Input: part model. Units: mm. Frame: model coordinates. Give positions to 0.01 mm unless a question says otherwise; leave off trailing zeros. Loops run counter-clockwise (first coordinate to the right, second up) from the corner with the lowest first, then second, coordinate; pieces in that order, holes last. Notation, with made-up numbers: M -33,-28 L 7,-28 A21 ccw 7,11 Z; hole C 49.25,77 d4. An arc over 180 degrees is marked long. One line per item, written item: value. Start each with the question number.
(1) Pin query (flat end, axial travel): P1, Ø1.1, axis at x = -2.5, z = 2, coming from the +Y side; P2, Ø1.5, axis at x = 206, z = 4, coming from the -Y side. Return the tip coordinate at first contact, or that it passes through.
(2) Ray query, line 1 along X through (y, z) = (-26.5, 2); line 2 along X through (y, z) = (41, 1); line 3 along X through (y, z) = (13, 1) (1 decimal). Return the intervals inside material, ascending. Write a range as from..to.
(3) Section A-A on z = 3. State how many separate pieces and enclosed holes the cut face has, plus the area to 3 significant figures.
(4) Section B-B on y = 57.5. Output: boundary loops of the cut face in (x, z).
```python
from build123d import *

# Parameters (mm, degrees)
SKETCH1_W             = 393.065
SKETCH1_H             = 127
BOSS_EXTRUDE1_DEPTH   = 6.35
SKETCH2_W             = 76.2
SKETCH2_H             = 25.654
CUT_EXTRUDE1_DEPTH    = 6.35
CUT_EXTRUDE2_DEPTH    = 6.35
LPATTERN1_COUNT       = 5
LPATTERN1_PITCH       = 22.225
BOSS_EXTRUDE2_DEPTH   = 6.35
LPATTERN2_COUNT       = 5
LPATTERN2_PITCH       = 22.225
BOSS_EXTRUDE3_DEPTH   = 6.35
BOSS_EXTRUDE3_2_DEPTH = 6.35
LPATTERN4_COUNT       = 3
LPATTERN4_PITCH       = 111.252
SKETCH14_W            = 50.8
SKETCH14_H            = 6.35
CUT_EXTRUDE3_DEPTH    = 6.35
SKETCH16_W            = 50.8
SKETCH16_H            = 6.35
CUT_EXTRUDE4_DEPTH    = 6.35
SKETCH19_W            = 47.8155
SKETCH19_H            = 6.35
CUT_EXTRUDE5_DEPTH    = 6.35


with BuildPart() as part:
    # Sketch1 → Boss-Extrude1 (new body)
    with BuildSketch(Plane.XY):
        Rectangle(SKETCH1_W, SKETCH1_H)
    extrude(amount=BOSS_EXTRUDE1_DEPTH)

    # Sketch2 → Cut-Extrude1 (cut)
    with BuildSketch(Plane.XY.offset(6.35)):
        with Locations((2.7305, -25.273)):
            Rectangle(SKETCH2_W, SKETCH2_H)
    extrude(amount=-CUT_EXTRUDE1_DEPTH, mode=Mode.SUBTRACT)

    # Sketch3 → Cut-Extrude2 (cut)
    with BuildSketch(Plane.XY.offset(6.35)):
        Polygon((-196.5325, 47.625), (-190.1825, 47.625), (-190.1825, 51.181), (-185.1025, 51.181), (-185.1025, 37.719), (-190.1825, 37.719), (-190.1825, 41.275), (-196.5325, 41.275), align=None)
    cut_extrude2 = extrude(amount=-CUT_EXTRUDE2_DEPTH, mode=Mode.SUBTRACT)

    # LPattern1: Cut-Extrude2 ×5
    with Locations(*[(0, -i * LPATTERN1_PITCH, 0) for i in range(1, LPATTERN1_COUNT)]):
        add(cut_extrude2, mode=Mode.SUBTRACT)


with BuildPart() as body_2:
    # Sketch4 → Boss-Extrude2 (new body)
    with BuildSketch(Plane.XY.offset(6.35)):
        Polygon((196.5325, 47.498), (202.8825, 47.498), (202.8825, 51.054), (207.9625, 51.054), (207.9625, 37.592), (202.8825, 37.592), (202.8825, 41.148), (196.5325, 41.148), align=None)
    boss_extrude2 = extrude(amount=-BOSS_EXTRUDE2_DEPTH)


with BuildPart() as lpattern2_1:
    # LPattern2: pattern copy
    add(boss_extrude2.moved(Location(Vector(0, -1, 0) * (1 * LPATTERN2_PITCH))))


with BuildPart() as lpattern2_2:
    # LPattern2: pattern copy
    add(boss_extrude2.moved(Location(Vector(0, -1, 0) * (2 * LPATTERN2_PITCH))))


with BuildPart() as lpattern2_3:
    # LPattern2: pattern copy
    add(boss_extrude2.moved(Location(Vector(0, -1, 0) * (3 * LPATTERN2_PITCH))))


with BuildPart() as lpattern2_4:
    # LPattern2: pattern copy
    add(boss_extrude2.moved(Location(Vector(0, -1, 0) * (4 * LPATTERN2_PITCH))))


with BuildPart() as body_2_1:
    add(body_2.part)

    # Combine1: union part, LPattern2_1, LPattern2_2, LPattern2_3, LPattern2_4
    add(part.part)
    add(lpattern2_1.part)
    add(lpattern2_2.part)
    add(lpattern2_3.part)
    add(lpattern2_4.part)


with BuildPart() as body_2_2:
    # Sketch12 → Boss-Extrude3 (new body)
    with BuildSketch(Plane.XY.offset(6.35)):
        Polygon((-196.5325, 81.5), (-196.5325, 63.5), (-112.832500014, 63.5), (-112.832500014, 65.5), (-113.832500014, 65.5), (-113.832500014, 67.5), (-112.832500014, 67.5), (-112.832500014, 75.5), (-120.3325, 75.5), (-120.3325, 81.5), align=None)
    boss_extrude3 = extrude(amount=-BOSS_EXTRUDE3_DEPTH)


with BuildPart() as body_3:
    # Sketch12 → Boss-Extrude3 2 (new body)
    with BuildSketch(Plane.XY.offset(6.35)):
        Polygon((-109.832500014, 65.5), (-109.832500014, 63.5), (-26.132500014, 63.5), (-26.132500014, 81.5), (-102.332500014, 81.5), (-102.332500014, 75.5), (-109.832500014, 75.5), (-109.832500014, 67.5), (-108.832500014, 67.5), (-108.832500014, 65.5), align=None)
    boss_extrude3_2 = extrude(amount=-BOSS_EXTRUDE3_2_DEPTH)


with BuildPart() as lpattern4_1:
    # LPattern4: pattern copy
    add(boss_extrude3.moved(Location(Vector(1, 0, 0) * (1 * LPATTERN4_PITCH))))


with BuildPart() as lpattern4_2:
    # LPattern4: pattern copy
    add(boss_extrude3.moved(Location(Vector(1, 0, 0) * (2 * LPATTERN4_PITCH))))


with BuildPart() as lpattern4_3:
    # LPattern4: pattern copy
    add(boss_extrude3_2.moved(Location(Vector(1, 0, 0) * (1 * LPATTERN4_PITCH))))


with BuildPart() as lpattern4_4:
    # LPattern4: pattern copy
    add(boss_extrude3_2.moved(Location(Vector(1, 0, 0) * (2 * LPATTERN4_PITCH))))


with BuildPart() as body_2_2_1:
    add(body_2_2.part)

    # Combine2: union body 3, LPattern4_3, LPattern4_1, LPattern4_2, LPattern4_4, body 2
    add(body_3.part)
    add(lpattern4_3.part)
    add(lpattern4_1.part)
    add(lpattern4_2.part)
    add(lpattern4_4.part)
    add(body_2_1.part)

    # Sketch14 → Cut-Extrude3 (cut)
    with BuildSketch(Plane.XY.offset(6.35)):
        with Locations((2.7305, 16.129)):
            Rectangle(SKETCH14_W, SKETCH14_H)
    extrude(amount=-CUT_EXTRUDE3_DEPTH, mode=Mode.SUBTRACT)

    # Sketch16 → Cut-Extrude4 (cut)
    with BuildSketch(Plane.XY.offset(6.35)):
        with Locations((129.7305, 16.129)):
            Rectangle(SKETCH16_W, SKETCH16_H)
    extrude(amount=-CUT_EXTRUDE4_DEPTH, mode=Mode.SUBTRACT)

    # Sketch19 → Cut-Extrude5 (cut)
    with BuildSketch(Plane.XY.offset(6.35)):
        with Locations((-122.77725, 16.129)):
            Rectangle(SKETCH19_W, SKETCH19_H)
    extrude(amount=-CUT_EXTRUDE5_DEPTH, mode=Mode.SUBTRACT)


solid = body_2_2_1.part
```
Output values:
1. P1: stops at y = 75.5
1. P2: stops at y = -51.31
2. line 1: x = -196.53..-190.18, -185.1..-35.37, 40.83..196.53, 202.88..207.96
2. line 2: x = -196.53..-190.18, -185.1..196.53, 202.88..207.96
2. line 3: x = -196.5..-146.7, -98.9..-22.7, 28.1..104.3, 155.1..196.5
3. separate pieces: 1
3. enclosed holes: 4
3. area: 53,600 mm²
4. outline: M -196.53,0 L 196.53,0 L 196.53,6.35 L -196.53,6.35 Z
